The listing builds one solid part. Answer for the finished solid, in the listing's coordinates (mm). A direction names the side the tool comes from. Give positions to 0.01 mm unless a question says otherwise; leave off trailing zeros. Loops run counter-clockwise (first coordinate to the right, second up) from the corner with the lowest first, then second, coordinate; pieces in that order, holes last. Notation, with made-up numbers: (20.25, 75) - (77.25, 75) arc R19 ccw to (77.25, 91) - close; hole circle Ø6 at (46.5, -23). An arc over 180 degrees is marked (long way). One line per item, written item: value. Start each with the question number.
from build123d import *

# Parameters (mm, degrees)
F0_R     = 2
F1_DEPTH = 1
F2_DEPTH = 1.5


with BuildPart() as f1:
    # F0 (on Top) → F1 (new body, symmetric)
    with BuildSketch(Plane.XY):
        Polygon((-9, -9), (9, -9), (9, 2), (5, 2), (5, 6), (-5, 6), (-5, 2), (-9, 2), align=None)
        Circle(F0_R, mode=Mode.SUBTRACT)
    extrude(amount=F1_DEPTH, both=True)

    # F0 (on Top) → F2 (join, symmetric)
    with BuildSketch(Plane.XY):
        Circle(F0_R)
    extrude(amount=F2_DEPTH, both=True)


solid = f1.part
1. A cutting plane is placed at B-B (z = -0.4). Determine the outline of the cut face in (x, y), plus the area to 3 significant figures.
2. Find the intervals of material crossed by L1, parallel to Y at x = 5.75, z = -0.85; L2, parallel to Z at x = -4.5, y = -0.5; L3, parallel to X at y = 4.25, z = 0.25, in increasing order. Write a range as [from, to].
3. A cutting plane is placed at D-D (y = -6). Determine the outline of the cut face in (x, z).
4. For faces 1 (the cylindrical face through (-0.434, -1.952, -1.246)), 2 (the flat face through (5, 4, 0)), 3 (the flat face through (-7, 2, 0)), determine the directions among +Z, -Z, +X, -X, +Y, -Y from which every point of the face is accessible in a straight line to the end or side of a thin tool.
5. A cutting plane is placed at C-C (x = 0). Determine the outline of the cut face in (y, z).
6. Flat-ended cylindrical pins translate along their axes: pin 1 (1.5 mm diameter, centred on x = -7, y = -2, fed in from +Z); pin 2 (0.6 mm diameter, centred on y = 4, z = 0.5, fed in from +X); pin 3 (4 mm diameter, centred on x = 4.5, y = -0.5, fed in from -Z). Find the tip coordinate at first contact, or state that the pin passes through.
7. A cutting plane is placed at A-A (y = 0). Determine the outline of the cut face in (x, z), plus the area to 3 significant figures.
Results below:
1. outline: (-9, -9) - (9, -9) - (9, 2) - (5, 2) - (5, 6) - (-5, 6) - (-5, 2) - (-9, 2) - close
1. area: 238 mm^2
2. L1: y = [-9, 2]
2. L2: z = [-1, 1]
2. L3: x = [-5, 5]
3. outline: (-9, -1) - (9, -1) - (9, 1) - (-9, 1) - close
4. face 1: -Z
4. face 2: +Z, -Z, +X, +Y
4. face 3: +Z, -Z, -X, +Y
5. outline: (-9, -1) - (-2, -1) - (-2, -1.5) - (2, -1.5) - (2, -1) - (6, -1) - (6, 1) - (2, 1) - (2, 1.5) - (-2, 1.5) - (-2, 1) - (-9, 1) - close
6. pin 1: stops at z = 1
6. pin 2: stops at x = 5
6. pin 3: stops at z = -1
7. outline: (-9, -1) - (-2, -1) - (-2, -1.5) - (2, -1.5) - (2, -1) - (9, -1) - (9, 1) - (2, 1) - (2, 1.5) - (-2, 1.5) - (-2, 1) - (-9, 1) - close
7. area: 40.0 mm^2
